```python
from build123d import *

# Parameters (mm, degrees)
F0_W     = 25
F0_H     = 35
F0_R     = 1.5
F0_R_2   = 5
F1_DEPTH = 3
F2_SIZE  = 5


with BuildPart() as f1:
    # F0 (on Front) → F1 (new body)
    with BuildSketch(Plane.XZ):
        with Locations((0, 5.5)):
            Rectangle(F0_W, F0_H)
        with Locations((-8, 0)):
            Circle(F0_R, mode=Mode.SUBTRACT)
        with Locations((0, -8)):
            Circle(F0_R, mode=Mode.SUBTRACT)
        Circle(F0_R_2, mode=Mode.SUBTRACT)
        with Locations((8, 0)):
            Circle(F0_R, mode=Mode.SUBTRACT)
        with Locations((-7.5, 18)):
            Circle(F0_R, mode=Mode.SUBTRACT)
        with Locations((0, 8)):
            Circle(F0_R, mode=Mode.SUBTRACT)
        with Locations((7.5, 18)):
            Circle(F0_R, mode=Mode.SUBTRACT)
    extrude(amount=F1_DEPTH)

    # F2
    f2_edges = [f1.edges().sort_by_distance(p)[0] for p in [
        (-12.5, -1.5, -12),
        (12.5, -1.5, -12),
    ]]
    chamfer(f2_edges, length=F2_SIZE)


solid = f1.part
```
Can you work these out from the model? Positions are in its coordinate system, mm. Give positions to 0.01 mm unless a question says otherwise; leave off trailing zeros. Loops run counter-clockwise (first coordinate to the right, second up) from the corner with the lowest first, then second, coordinate; pieces in that order, holes last. Notation, with made-up numbers: M 35,-18 L 46,-18 A21 ccw 46,-9 Z; hole C 5,-7 d4. An arc over 180 degrees is marked long. One line per item, written item: value.
(1) Suppose I cut it at A-A on x = 4. List the corners of the cut face in (y, z) for me.
Returned:
outline: M -3,-12 L 0,-12 L 0,-3 L -3,-3 Z; M -3,3 L 0,3 L 0,23 L -3,23 Z
(2) Suppose I cut it at D-D on y = -2.2. List the corners of the cut face in (x, z) for me, plus the area to 3 significant figures.
Returned:
outline: M -12.5,-7 L -7.5,-12 L 7.5,-12 L 12.5,-7 L 12.5,23 L -12.5,23 Z; hole C -8,0 d3; hole C -7.5,18 d3; hole C 0,0 d10; hole C 0,-8 d3; hole C 0,8 d3; hole C 7.5,18 d3; hole C 8,0 d3
area: 729 mm^2
(3) Suppose I cut it at C-C on x = -8. List the corners of the cut face in (y, z) for me, plus the area to 3 significant figures.
Returned:
outline: M -3,-11.5 L 0,-11.5 L 0,-1.5 L -3,-1.5 Z; M -3,1.5 L 0,1.5 L 0,16.59 L -3,16.59 Z; M -3,19.41 L 0,19.41 L 0,23 L -3,23 Z
area: 86.0 mm^2
(4) Will this pin go through, and if not, where does the flat tip stop? pin 1 (3 mm diameter, centred on x = -1, z = -2.5, fed in from -Y).
Returned:
pin 1: through
(5) We'd pull the mould along X, two halves only. Please class faces 1 (the face through (12.5, -1, 8)), 2 (the face through (0, -3, 6)), 3 (the face through (-0.325, -1.479, -9.464)), 4 (the face through (-9.5, -1.48, 0.07)): released by +X, released by -X, zero draft, split by the parting line, or undercut.
Returned:
face 1: released by +X
face 2: zero draft
face 3: undercut
face 4: undercut
(6) I need wall thicknesses on line 1 (Z direction, x = 0, y = -1.45); line 2 (Z direction, x = -8, y = -2); line 3 (Z direction, x = 7.75, y = -1). Which ranges of each line are inside material? Lowest first, please.
Returned:
line 1: -12 to -9.5, -6.5 to -5, 5 to 6.5, 9.5 to 23
line 2: -11.5 to -1.5, 1.5 to 16.59, 19.41 to 23
line 3: -11.75 to -1.48, 1.48 to 16.52, 19.48 to 23
(7) Suppose I cut it at B-B on z = 8. List the corners of the cut face in (x, y) for me, plus the area to 3 significant figures.
Returned:
outline: M -12.5,-3 L -1.5,-3 L -1.5,0 L -12.5,0 Z; M 1.5,-3 L 12.5,-3 L 12.5,0 L 1.5,0 Z
area: 66.0 mm^2
